from build123d import *

# Parameters (mm, degrees)
SKETCH1_R                   = 5
SKETCH1_R_2                 = 4
SKETCH1_R_3                 = 14.5
SKETCH1_R_4                 = 9
SKETCH1_R_5                 = 13.72
SKETCH1_R_6                 = 3.22
SKETCH1_R_7                 = 5.5
BOSS_EXTRUDE1_DEPTH         = 36
M8_TAPPED_HOLE2_D           = 6.8
M8_TAPPED_HOLE2_CSINK_D     = 8.05
M8_TAPPED_HOLE2_CSINK_ANGLE = 90
CUT_EXTRUDE1_DEPTH          = 8
SKETCH1_4_R                 = 9
SKETCH1_4_R_2               = 5.5
CUT_EXTRUDE2_DEPTH          = 16
CUT_EXTRUDE3_START          = -8
SKETCH1_5_R                 = 4
SKETCH1_5_R_2               = 3.22
SKETCH1_5_R_3               = 14.5
SKETCH1_5_R_4               = 13.72
CUT_EXTRUDE3_DEPTH          = 117.583305463
M8_TAPPED_HOLE1_D           = 6.8
M8_TAPPED_HOLE1_DEPTH       = 12.957073895
M8_TAPPED_HOLE1_TIP         = 2.042926105


with BuildPart() as part:
    # Sketch1 → Boss-Extrude1 (new body)
    # profile 1 of 10: a face of its own
    with BuildSketch(Plane(origin=(0, 0, 0), x_dir=(1, 0, 0), z_dir=(0, 1, 0))):
        Polygon((100, -55), (100, 55), (90, 65), (-90, 65), (-100, 55), (-100, -55), (-90, -65), (90, -65), align=None)
        with Locations(Location((-65, 45, 0), (0, 0, 270))):
            Circle(SKETCH1_R, mode=Mode.SUBTRACT)
        with Locations(Location((55, -45, 0), (0, 0, 270))):
            Circle(SKETCH1_R, mode=Mode.SUBTRACT)
        with Locations((32.483339502, 13)):
            Circle(SKETCH1_R_2, mode=Mode.SUBTRACT)
        with Locations((55, -26)):
            Circle(SKETCH1_R_2, mode=Mode.SUBTRACT)
        with Locations((77.516660498, 13)):
            Circle(SKETCH1_R_2, mode=Mode.SUBTRACT)
        with Locations((55, 0)):
            Circle(SKETCH1_R_3, mode=Mode.SUBTRACT)
        with Locations((80, 45)):
            Circle(SKETCH1_R_4, mode=Mode.SUBTRACT)
        with Locations((-80, 45)):
            Circle(SKETCH1_R_4, mode=Mode.SUBTRACT)
        with Locations((80, -45)):
            Circle(SKETCH1_R_4, mode=Mode.SUBTRACT)
        with Locations((-80, -45)):
            Circle(SKETCH1_R_4, mode=Mode.SUBTRACT)
        with BuildLine():
            ThreePointArc((-80.507041555, 25.5), (-84.837168574, 23), (-84.837168574, 18))
            Line((-84.837168574, 18), (-49.330127019, -43.5))
            ThreePointArc((-49.330127019, -43.5), (-45, -46), (-40.669872981, -43.5))
            Line((-40.669872981, -43.5), (-5.162831426, 18))
            ThreePointArc((-5.162831426, 18), (-5.162831426, 23), (-9.492958445, 25.5))
            Line((-9.492958445, 25.5), (-80.507041555, 25.5))
        make_face(mode=Mode.SUBTRACT)
    # profile 2 of 10: a face of its own
    with BuildSketch(Plane(origin=(0, 0, 0), x_dir=(1, 0, 0), z_dir=(0, 1, 0))):
        with BuildLine():
            Line((-9.492958445, 25.5), (-80.507041555, 25.5))
            ThreePointArc((-80.507041555, 25.5), (-84.837168574, 23), (-84.837168574, 18))
            Line((-84.837168574, 18), (-49.330127019, -43.5))
            ThreePointArc((-49.330127019, -43.5), (-45, -46), (-40.669872981, -43.5))
            Line((-40.669872981, -43.5), (-5.162831426, 18))
            ThreePointArc((-5.162831426, 18), (-5.162831426, 23), (-9.492958445, 25.5))
        make_face()
        with BuildLine():
            ThreePointArc((-6.02885683, 18.5), (-6.02885683, 22.5), (-9.492958445, 24.5))
            Line((-9.492958445, 24.5), (-80.507041555, 24.5))
            ThreePointArc((-80.507041555, 24.5), (-83.97114317, 22.5), (-83.97114317, 18.5))
            Line((-83.97114317, 18.5), (-48.464101615, -43))
            ThreePointArc((-48.464101615, -43), (-45, -45), (-41.535898385, -43))
            Line((-41.535898385, -43), (-6.02885683, 18.5))
        make_face(mode=Mode.SUBTRACT)
    # profile 3 of 10: a face of its own
    with BuildSketch(Plane(origin=(0, 0, 0), x_dir=(1, 0, 0), z_dir=(0, 1, 0))):
        with Locations((55, 0)):
            Circle(SKETCH1_R_3)
        with Locations(Location((55, 0, 0), (0, 0, 270))):
            Circle(SKETCH1_R_5, mode=Mode.SUBTRACT)
    # profile 4 of 10: a face of its own
    with BuildSketch(Plane(origin=(0, 0, 0), x_dir=(1, 0, 0), z_dir=(0, 1, 0))):
        with Locations((32.483339502, 13)):
            Circle(SKETCH1_R_2)
        with Locations(Location((32.483339502, 13, 0), (0, 0, 270))):
            Circle(SKETCH1_R_6, mode=Mode.SUBTRACT)
    # profile 5 of 10: a face of its own
    with BuildSketch(Plane(origin=(0, 0, 0), x_dir=(1, 0, 0), z_dir=(0, 1, 0))):
        with Locations((77.516660498, 13)):
            Circle(SKETCH1_R_2)
        with Locations(Location((77.516660498, 13, 0), (0, 0, 270))):
            Circle(SKETCH1_R_6, mode=Mode.SUBTRACT)
    # profile 6 of 10: a face of its own
    with BuildSketch(Plane(origin=(0, 0, 0), x_dir=(1, 0, 0), z_dir=(0, 1, 0))):
        with Locations((55, -26)):
            Circle(SKETCH1_R_2)
        with Locations(Location((55, -26, 0), (0, 0, 270))):
            Circle(SKETCH1_R_6, mode=Mode.SUBTRACT)
    # profile 7 of 10: a face of its own
    with BuildSketch(Plane(origin=(0, 0, 0), x_dir=(1, 0, 0), z_dir=(0, 1, 0))):
        with Locations((80, -45)):
            Circle(SKETCH1_R_4)
        with Locations(Location((80, -45, 0), (0, 0, 270))):
            Circle(SKETCH1_R_7, mode=Mode.SUBTRACT)
    # profile 8 of 10: a face of its own
    with BuildSketch(Plane(origin=(0, 0, 0), x_dir=(1, 0, 0), z_dir=(0, 1, 0))):
        with Locations((80, 45)):
            Circle(SKETCH1_R_4)
        with Locations(Location((80, 45, 0), (0, 0, 270))):
            Circle(SKETCH1_R_7, mode=Mode.SUBTRACT)
    # profile 9 of 10: a face of its own
    with BuildSketch(Plane(origin=(0, 0, 0), x_dir=(1, 0, 0), z_dir=(0, 1, 0))):
        with Locations((-80, 45)):
            Circle(SKETCH1_R_4)
        with Locations(Location((-80, 45, 0), (0, 0, 270))):
            Circle(SKETCH1_R_7, mode=Mode.SUBTRACT)
    # profile 10 of 10: a face of its own
    with BuildSketch(Plane(origin=(0, 0, 0), x_dir=(1, 0, 0), z_dir=(0, 1, 0))):
        with Locations((-80, -45)):
            Circle(SKETCH1_R_4)
        with Locations(Location((-80, -45, 0), (0, 0, 270))):
            Circle(SKETCH1_R_7, mode=Mode.SUBTRACT)
    extrude(amount=-BOSS_EXTRUDE1_DEPTH)

    # M8 Tapped Hole2 (through all)
    with Locations(Plane(origin=(0, 0, 0), x_dir=(1, 0, 0), z_dir=(0, 1, 0))):
        with Locations((-45, 45), (55, 45)):
            CounterSinkHole(M8_TAPPED_HOLE2_D / 2, M8_TAPPED_HOLE2_CSINK_D / 2, counter_sink_angle=M8_TAPPED_HOLE2_CSINK_ANGLE)

    # Sketch1_3 → Cut-Extrude1 (cut)
    with BuildSketch(Plane(origin=(0, 0, 0), x_dir=(1, 0, 0), z_dir=(0, 1, 0))):
        with BuildLine():
            Line((-9.492958445, 25.5), (-80.507041555, 25.5))
            ThreePointArc((-80.507041555, 25.5), (-84.837168574, 23), (-84.837168574, 18))
            Line((-84.837168574, 18), (-49.330127019, -43.5))
            ThreePointArc((-49.330127019, -43.5), (-45, -46), (-40.669872981, -43.5))
            Line((-40.669872981, -43.5), (-5.162831426, 18))
            ThreePointArc((-5.162831426, 18), (-5.162831426, 23), (-9.492958445, 25.5))
        make_face()
        with BuildLine():
            ThreePointArc((-6.02885683, 18.5), (-6.02885683, 22.5), (-9.492958445, 24.5))
            Line((-9.492958445, 24.5), (-80.507041555, 24.5))
            ThreePointArc((-80.507041555, 24.5), (-83.97114317, 22.5), (-83.97114317, 18.5))
            Line((-83.97114317, 18.5), (-48.464101615, -43))
            ThreePointArc((-48.464101615, -43), (-45, -45), (-41.535898385, -43))
            Line((-41.535898385, -43), (-6.02885683, 18.5))
        make_face(mode=Mode.SUBTRACT)
    extrude(amount=-CUT_EXTRUDE1_DEPTH, mode=Mode.SUBTRACT)

    # Sketch1_4 → Cut-Extrude2 (cut)
    # profile 1 of 4: a face of its own
    with BuildSketch(Plane(origin=(0, 0, 0), x_dir=(1, 0, 0), z_dir=(0, 1, 0))):
        with Locations(Location((-80, 45, 0), (0, 0, 270))):
            Circle(SKETCH1_4_R)
        with Locations(Location((-80, 45, 0), (0, 0, 270))):
            Circle(SKETCH1_4_R_2, mode=Mode.SUBTRACT)
    # profile 2 of 4: a face of its own
    with BuildSketch(Plane(origin=(0, 0, 0), x_dir=(1, 0, 0), z_dir=(0, 1, 0))):
        with Locations(Location((80, 45, 0), (0, 0, 270))):
            Circle(SKETCH1_4_R)
        with Locations(Location((80, 45, 0), (0, 0, 270))):
            Circle(SKETCH1_4_R_2, mode=Mode.SUBTRACT)
    # profile 3 of 4: a face of its own
    with BuildSketch(Plane(origin=(0, 0, 0), x_dir=(1, 0, 0), z_dir=(0, 1, 0))):
        with Locations(Location((80, -45, 0), (0, 0, 270))):
            Circle(SKETCH1_4_R)
        with Locations(Location((80, -45, 0), (0, 0, 270))):
            Circle(SKETCH1_4_R_2, mode=Mode.SUBTRACT)
    # profile 4 of 4: a face of its own
    with BuildSketch(Plane(origin=(0, 0, 0), x_dir=(1, 0, 0), z_dir=(0, 1, 0))):
        with Locations(Location((-80, -45, 0), (0, 0, 270))):
            Circle(SKETCH1_4_R)
        with Locations(Location((-80, -45, 0), (0, 0, 270))):
            Circle(SKETCH1_4_R_2, mode=Mode.SUBTRACT)
    extrude(amount=-CUT_EXTRUDE2_DEPTH, mode=Mode.SUBTRACT)

    # Sketch1_5 → Cut-Extrude3 (cut, through all)
    # profile 1 of 5: a face of its own
    with BuildSketch(Plane(origin=(0, 0, 0), x_dir=(1, 0, 0), z_dir=(0, 1, 0)).offset(CUT_EXTRUDE3_START)):
        with Locations(Location((77.516660498, 13, 0), (0, 0, 270))):
            Circle(SKETCH1_5_R)
        with Locations(Location((77.516660498, 13, 0), (0, 0, 270))):
            Circle(SKETCH1_5_R_2, mode=Mode.SUBTRACT)
    # profile 2 of 5: a face of its own
    with BuildSketch(Plane(origin=(0, 0, 0), x_dir=(1, 0, 0), z_dir=(0, 1, 0)).offset(CUT_EXTRUDE3_START)):
        with Locations(Location((32.483339502, 13, 0), (0, 0, 270))):
            Circle(SKETCH1_5_R)
        with Locations(Location((32.483339502, 13, 0), (0, 0, 270))):
            Circle(SKETCH1_5_R_2, mode=Mode.SUBTRACT)
    # profile 3 of 5: a face of its own
    with BuildSketch(Plane(origin=(0, 0, 0), x_dir=(1, 0, 0), z_dir=(0, 1, 0)).offset(CUT_EXTRUDE3_START)):
        with Locations(Location((55, -26, 0), (0, 0, 270))):
            Circle(SKETCH1_5_R)
        with Locations(Location((55, -26, 0), (0, 0, 270))):
            Circle(SKETCH1_5_R_2, mode=Mode.SUBTRACT)
    # profile 4 of 5: a face of its own
    with BuildSketch(Plane(origin=(0, 0, 0), x_dir=(1, 0, 0), z_dir=(0, 1, 0)).offset(CUT_EXTRUDE3_START)):
        with Locations(Location((55, 0, 0), (0, 0, 270))):
            Circle(SKETCH1_5_R_3)
        with Locations(Location((55, 0, 0), (0, 0, 270))):
            Circle(SKETCH1_5_R_4, mode=Mode.SUBTRACT)
    # profile 5 of 5: a face of its own
    with BuildSketch(Plane(origin=(0, 0, 0), x_dir=(1, 0, 0), z_dir=(0, 1, 0)).offset(CUT_EXTRUDE3_START)):
        with Locations(Location((55, 0, 0), (0, 0, 270))):
            Circle(SKETCH1_5_R_4)
    extrude(amount=-CUT_EXTRUDE3_DEPTH, mode=Mode.SUBTRACT)

    # M8 Tapped Hole1
    with Locations(Plane.XY.offset(65)):
        with Locations((-60, -15), (50, -15)):
            Hole(M8_TAPPED_HOLE1_D / 2, depth=M8_TAPPED_HOLE1_DEPTH)
            with Locations((0, 0, -(M8_TAPPED_HOLE1_DEPTH + M8_TAPPED_HOLE1_TIP / 2))):  # 118° drill point
                Cone(0, M8_TAPPED_HOLE1_D / 2, M8_TAPPED_HOLE1_TIP, mode=Mode.SUBTRACT)


solid = part.part
Part model, mm, in its own coordinate system. A direction names the side the tool comes from. Round coordinates to 2 decimals unless told otherwise and drop trailing zeros. Write each loop counter-clockwise with the first axis right and the second up, starting at its lowest first coordinate (ties: lowest second). Pieces come first, ordered by that corner, then holes. Notation, with made-up numbers: (68, 48.5) - (82, 48.5) arc R18 cw to (82, 61.5) - close; hole circle Ø5 at (-21, 80.25). An arc over 180 degrees is marked (long way). Use CSV: the item, a comma, the result in double quotes.
Item 1: Slice it at C-C, the plane y = -3.5. Count the separate pieces of the cut face and the enclosed holes in it, then the cut area to 3 significant figures.
Results list:
separate pieces,"1"
enclosed holes,"13"
area,"20,500 mm²"
Item 2: Slice it at D-D, the plane z = 57. Write the cut outline in (x, y), then the cut area to 3 significant figures.
Results list:
outline,"(-98, -36) - (98, -36) - (98, 0) - (-98, 0) - close; hole circle Ø6.8 at (-60, -15); hole circle Ø6.8 at (50, -15)"
area,"6,980 mm²"
Item 3: Flat gauge pins, fed straight in: P1, Ø4, axis at x = 55, z = -45, coming from the -Y side; P2, Ø5.5, axis at x = -84, z = -47.5, coming from the +Y side. Where does each tip first touch, or does it go through?
Results list:
P1,"passes through"
P2,"stops at y = -16"
Item 4: Pull direction X, two halves, no side cores. Call faces 1 (the cylindrical face through (81.483, -21.804, -13.521)), 2 (the flat face through (-1, 0, -1)), 3 (the flat face through (100, -18, 1)), 4 (the flat face through (57, -8, 23)): pulls with the +X half, pulls with the -X half, needs draft (parallel to the pull), parting line crosses it, or undercut.
Results list:
face 1,"undercut"
face 2,"needs draft"
face 3,"pulls with the +X half"
face 4,"undercut"
Item 5: Slice it at B-B, the plane z = 32.5. Write the cut outline in (x, y).
Results list:
outline,"(-100, -36) - (-54.53, -36) - (-54.53, -8) - (-55.68, -8) - (-55.68, 0) - (-100, 0) - close; (-35.47, -36) - (100, -36) - (100, 0) - (-34.32, 0) - (-34.32, -8) - (-35.47, -8) - close"
Item 6: Slice it at A-A, the plane x = -45. Write the cut outline in (y, z) (3 decimals), then the cut area to 3 significant figures.
Results list:
outline,"(-36, -65) - (0, -65) - (0, -49.025) - (-0.625, -48.4) - (-36, -48.4) - close; (-36, -41.6) - (-0.625, -41.6) - (0, -40.975) - (0, -25.5) - (-8, -25.5) - (-8, -24.5) - (-36, -24.5) - close; (-36, 45) - (-8, 45) - (-8, 46) - (0, 46) - (0, 65) - (-36, 65) - close"
area,"1,920 mm²"
Item 7: Tool access for faces 5 (the cylindrical face through (40.845, -21.804, -3.143)), 6 (the flat face through (-1, -36, -1)), 7 (the cylindrical face through (71.214, -7.888, -46.951)): list every direction of +Z, -Z, +X, -X, +Y, -Y with a clear straight run to the whole face (end or side of a thin tool).
Results list:
face 5,"-Y"
face 6,"+Z, -Z, +X, -X, -Y"
face 7,"+Y"
Item 8: Wall check: L1, parallel to X at y = -20, z = -45; L2, parallel to X at y = -5, z = 41.5; L3, parallel to X at y = -21.5, z = -1.5. Give the ranges that are in metal, low to high.
Results list:
L1,"x = -100 to -85.5, -74.5 to -70, -60 to -48.4, -41.6 to 51.6, 58.4 to 74.5, 85.5 to 100"
L2,"x = -100 to -88.29, -71.71 to -50.48, -39.52 to 51.43, 58.57 to 71.71, 88.29 to 100"
L3,"x = -100 to -74.16, -15.84 to 40.58, 69.42 to 100"
